The listing builds one solid part. Answer for the finished solid, in the listing's coordinates (mm). A direction names the side the tool comes from. Give positions to 0.01 mm unless a question says otherwise; leave off trailing zeros. Loops run counter-clockwise (first coordinate to the right, second up) from the corner with the lowest first, then second, coordinate; pieces in that order, holes last.
Item 1: Section C-C, the plane x = -5 is taken. Give the vertices of the cut face in (y, z).
Item 2: Section D-D, the plane z = -15 is taken. Give the vertices of the cut face in (x, y).
Item 3: Section B-B, the plane y = -0.35 is taken. Give the vertices of the cut face in (x, z), and give its area (3 significant figures).
Item 4: The mould has two halves that part along X. Classify faces 6 (the face through (0, 0, 6)), 7 (the face through (-16.67, 0.02, -10.82)), 8 (the face through (14.595, 0.021, -22.592)), 9 (the face through (4, 0, 5)): pulls with the +X half, pulls with the -X half, needs draft (parallel to the pull), parting line crosses it, or undercut.
Item 5: Each of these flat-tipped pins is pushed along its axis until it touches: pin 1 Ø1.5 at (x, y) = (14, -0.5) entering from +Z; pin 2 Ø1.5 at (y, z) = (0.5, 4.5) entering from +X. Where does it stop, or does it pass through?
Item 6: Section A-A, the plane x = 0 is taken. Give the vertices of the cut face in (y, z), and give its area (4 significant figures).
Item 7: A tool of negligible diameter and unlimited length cuts with its end or side. For faces 1 (the face through (13, 0, 0)), 2 (the face through (-14.997, 0.021, -11.554)), 3 (the face through (-8.579, 0, 4)), 4 (the face through (13.26, 0.02, -21.4)), 5 (the face through (-13.3, 0.02, -21.41)), from which of +Z, -Z, +X, -X, +Y, -Y can it reach the whole face along a straight path? Write none if from no direction.
Item 8: Consider line 1 along Z through (x, y) = (2.5, -1); line 2 along X through (y, z) = (-0.2, -21); line 3 along Z through (x, y) = (-6.5, -1.1). Determine where each line is inside the solid, lowest interval first.
from build123d import *

# Parameters (mm, degrees)
SKETCH1_R           = 7.65
SKETCH1_W           = 8
SKETCH1_H           = 3
BOSS_EXTRUDE1_DEPTH = 1.5


with BuildPart() as part:
    # Sketch1 → Boss-Extrude1 (new, symmetric)
    with BuildSketch(Plane(origin=(0, 0, 0), x_dir=(1, 0, 0), z_dir=(0, 1, 0))):
        with BuildLine():
            Line((-16.852566459, 9.790333805), (-16.852566459, 0))
            Line((-16.852566459, 0), (-8.578866459, 0))
            Line((-8.578866459, 0), (-8.578866459, -9))
            Line((-8.578866459, -9), (8.578866459, -9))
            Line((8.578866459, -9), (8.578866459, 0))
            Line((8.578866459, 0), (16.852566459, 0))
            Line((16.852566459, 0), (16.852566459, 9.790333805))
            Line((16.852566459, 9.790333805), (16.495088327, 11.817693036))
            Line((16.495088327, 11.817693036), (13.540665068, 11.296748503))
            Line((13.540665068, 11.296748503), (11.804183291, 21.144826033))
            Line((11.804183291, 21.144826033), (14.75860655, 21.665770566))
            Line((14.75860655, 21.665770566), (14.427433582, 23.543945803))
            ThreePointArc((14.427433582, 23.543945803), (0, 35.65), (-14.427433582, 23.543945803))
            Line((-14.427433582, 23.543945803), (-14.75860655, 21.665770566))
            Line((-14.75860655, 21.665770566), (-11.804183291, 21.144826033))
            Line((-11.804183291, 21.144826033), (-13.540665068, 11.296748503))
            Line((-13.540665068, 11.296748503), (-16.495088327, 11.817693036))
            Line((-16.495088327, 11.817693036), (-16.852566459, 9.790333805))
        make_face()
        with Locations((0, 21)):
            Circle(SKETCH1_R, mode=Mode.SUBTRACT)
        with Locations((0, -4.5)):
            Rectangle(SKETCH1_W, SKETCH1_H, mode=Mode.SUBTRACT)
    extrude(amount=BOSS_EXTRUDE1_DEPTH, both=True)


solid = part.part
Worked answers:
1. outline: (-1.5, -34.77) - (1.5, -34.77) - (1.5, -26.79) - (-1.5, -26.79) - close; (-1.5, -15.21) - (1.5, -15.21) - (1.5, 9) - (-1.5, 9) - close
2. outline: (-12.89, -1.5) - (-4.75, -1.5) - (-4.75, 1.5) - (-12.89, 1.5) - close; (4.75, -1.5) - (12.89, -1.5) - (12.89, 1.5) - (4.75, 1.5) - close
3. outline: (-16.85, -9.79) - (-16.5, -11.82) - (-13.54, -11.3) - (-11.8, -21.14) - (-14.76, -21.67) - (-14.43, -23.54) arc R14.65 ccw to (14.43, -23.54) - (14.76, -21.67) - (11.8, -21.14) - (13.54, -11.3) - (16.5, -11.82) - (16.85, -9.79) - (16.85, 0) - (8.58, 0) - (8.58, 9) - (-8.58, 9) - (-8.58, 0) - (-16.85, 0) - close; hole circle Ø15.3 at (0, -21); hole (-4, 3) - (4, 3) - (4, 6) - (-4, 6) - close
3. area: 910 mm2
4. face 6: undercut
4. face 7: pulls with the -X half
4. face 8: pulls with the +X half
4. face 9: undercut
5. pin 1: stops at z = 0
5. pin 2: stops at x = 8.58
6. outline: (-1.5, -35.65) - (1.5, -35.65) - (1.5, -28.65) - (-1.5, -28.65) - close; (-1.5, -13.35) - (1.5, -13.35) - (1.5, 3) - (-1.5, 3) - close; (-1.5, 6) - (1.5, 6) - (1.5, 9) - (-1.5, 9) - close
6. area: 79.05 mm2
7. face 1: +Z, +X, +Y, -Y
7. face 2: +Y, -Y
7. face 3: +Z, -X, +Y, -Y
7. face 4: +X, +Y, -Y
7. face 5: -X, +Y, -Y
8. line 1: z = -35.44 to -28.23, -13.77 to 3, 6 to 9
8. line 2: x = -11.83 to -7.65, 7.65 to 11.83
8. line 3: z = -34.13 to -25.03, -16.97 to 9
